```python
from build123d import *

# Parameters (mm, degrees)
SKETCH1_W           = 50.8
SKETCH1_H           = 254
BOSS_EXTRUDE1_DEPTH = 15.875
CHAMFER1_SIZE       = 25.4
CHAMFER1_SIZE2      = 12.7
SKETCH2_R           = 4.7625
CUT_EXTRUDE1_DEPTH  = 16.875
SKETCH3_W           = 38.1
SKETCH3_H           = 152.4
BOSS_EXTRUDE2_DEPTH = 15.875


with BuildPart() as part:
    # Sketch1 → Boss-Extrude1 (new body)
    with BuildSketch(Plane.XY):
        with Locations((25.4, 127)):
            Rectangle(SKETCH1_W, SKETCH1_H)
    extrude(amount=BOSS_EXTRUDE1_DEPTH)

    # Chamfer1
    chamfer1_edges = [part.edges().sort_by_distance(p)[0] for p in [
        (0, 0, 7.9375),
    ]]
    chamfer1_side = [part.faces().sort_by_distance(p)[0] for p in [
        (0, 127, 7.9375),
    ]]
    chamfer(chamfer1_edges, length=CHAMFER1_SIZE, length2=CHAMFER1_SIZE2, reference=chamfer1_side[0])

    # Sketch2 → Cut-Extrude1 (cut, through all)
    with BuildSketch(Plane.XY.offset(15.875)):
        with Locations((25.4, 25.4)):
            Circle(SKETCH2_R)
    extrude(amount=-CUT_EXTRUDE1_DEPTH, mode=Mode.SUBTRACT)

    # Sketch3 → Boss-Extrude2 (add)
    with BuildSketch(Plane.XY.offset(15.875)):
        with Locations((31.75, -76.2)):
            Rectangle(SKETCH3_W, SKETCH3_H)
    extrude(amount=-BOSS_EXTRUDE2_DEPTH)


solid = part.part
```
Read the model definition and answer for the solid it produces. Units are mm, in the model's axes. A direction names the side the tool comes from. Give positions to 0.01 mm unless a question says otherwise; leave off trailing zeros. Order: outer loops, then holes, each group sorted by start corner. A loop starts at its lowest first (then second) coordinate and runs counter-clockwise, first axis right, second up. Notation, with made-up numbers: (-7.5, -32) -> (17.5, -32) arc R19 ccw to (17.5, -24) -> close; hole circle Ø5 at (-24, -7). An arc over 180 degrees is marked (long way). One line per item, written item: value. Start each with the question number.
(1) Flat-ended cylindrical pins translate along their axes: P1, Ø3, axis at y = -87.5, z = 5, coming from the -X side; P2, Ø5, axis at y = 3.5, z = 5, coming from the -X side. Find the tip coordinate at first contact, or state that the pin passes through.
(2) The part is cut by section A-A (x = 25.4). Determine the outline of the cut face in (y, z) (1 decimal).
(3) The part is cut by section C-C (x = 4). Determine the outline of the cut face in (y, z) (3 decimals), and give its area (3 significant figures).
(4) Straight lines are drawn through the part: L1, parallel to Y at x = 25.4, z = 5.25; L2, parallel to X at y = -123.5, z = 6.5; L3, parallel to Y at x = 5, z = 2.5. For each, find the intervals that lie inside material, in ascending order.
(5) For a pull along Y with two mould halves and no side action, classify faces 3 (the cylindrical face through (27.96, 29.416, 8.049)), 4 (the flat face through (0, 138, 8)), 5 (the flat face through (25, 254, 8)) as released by +Y, released by -Y, zero draft, split by the parting line, or undercut.
(6) A tool of negligible diameter and unlimited length cuts with its end or side. For faces 1 (the flat face through (31, -152.4, 8)), 2 (the flat face through (12.7, -77, 8)), from which of +Z, -Z, +X, -X, +Y, -Y can it reach the whole face along a straight path? Write none if from no direction.
(7) The part is cut by section B-B (z = 7.5). Determine the outline of the cut face in (x, y) (1 decimal), and give its area (3 significant figures).
Taken from the geometry:
1. P1: x = 12.7
1. P2: x = 9.7
2. outline: (-152.4, 0) -> (20.6, 0) -> (20.6, 15.9) -> (-152.4, 15.9) -> close; (30.2, 0) -> (254, 0) -> (254, 15.9) -> (30.2, 15.9) -> close
3. outline: (17.4, 0) -> (254, 0) -> (254, 15.875) -> (17.4, 15.875) -> close
3. area: 3,760 mm^2
4. L1: -152.4 to 20.64, 30.16 to 254
4. L2: 12.7 to 50.8
4. L3: 15.4 to 254
5. face 3: undercut
5. face 4: zero draft
5. face 5: released by +Y
6. face 1: +Z, -Z, +X, -X, -Y
6. face 2: +Z, -Z, -X, -Y
7. outline: (0, 25.4) -> (12.7, 0) -> (12.7, -152.4) -> (50.8, -152.4) -> (50.8, 254) -> (0, 254) -> close; hole circle Ø9.5 at (25.4, 25.4)
7. area: 18,500 mm^2
